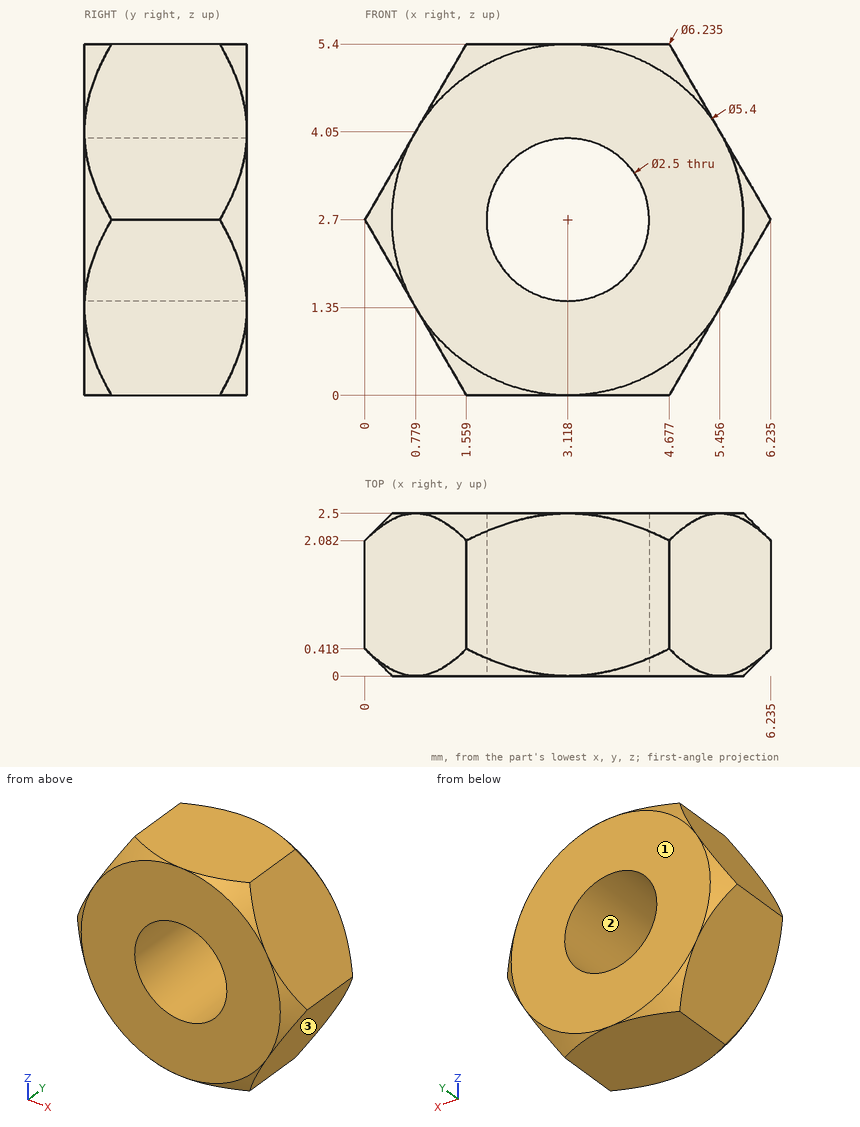
Check sheet for the drawn part. Datum: minimum x, y, z corner. Units: mm. Round coordinates to 2 decimals unless told otherwise and drop trailing zeros. Write each question's results on one line, items separated by ' | '. Start each with the question number.
Q1. Thickness scan on line 1 (Z direction, x = 2.75, y = 2.2) (1 decimal); line 2 (Z direction, x = 4, y = 0.3) (1 decimal); line 3 (X direction, y = 0.25, z = 3.7) (1 decimal). Record the ranges inside material, lowest first. Write a range as [from, to].
Q2. Release check for a two-part mould opening along Z. For the marked faces 1, 2 and 3 record: +Z half, -Z half, draft (parallel to the pull), parting line (faces both ways), or undercut.
Q3. Gauge pin test, flat ends, axial feed: P1, Ø3, axis at x = 3.12, z = 2.7, coming from the +Y side; P2, Ø1, axis at y = 0.5, z = 2, coming from the -X side (1 decimal). Record the tip position at first contact, or that the pin passes through.
Answers below:
1) line 1: z = [0, 1.5], [3.9, 5.4] | line 2: z = [0, 1.8], [3.6, 5.4] | line 3: x = [0.6, 2.4], [3.9, 5.7]
2) face 1: draft | face 2: undercut | face 3: -Z half
3) P1: stops at y = 2.5 | P2: stops at x = 0.1
